Read the model definition and answer for the solid it produces. Units are mm, in the model's axes. A direction names the side the tool comes from. Coordinates: 2 decimals unless noted, no trailing zeros. Order: outer loops, then holes, each group sorted by start corner. A loop starts at its lowest first (then second) coordinate and runs counter-clockwise, first axis right, second up. Notation, with made-up numbers: M 33.5,24 L 59.5,24 A11 ccw 59.5,32 Z; hole C 78.5,14 d2. An arc over 180 degrees is marked long. One line per question, with ' | ' between items. Start each with the question number.
1) A tool of negligible diameter and unlimited length cuts with its end or side. For faces 4 (the face through (-35.357, 48.514, -99.555)), 5 (the face through (-60.933, 18, -98)), 6 (the face through (-56.17, 5.03, -97.92)), from which of +Z, -Z, +X, -X, +Y, -Y can it reach the whole face along a straight path? Write none if from no direction.
2) Given P1, Ø1.6, axis at x = -35.53, z = -98.21, coming from the +Y side; P2, Ø1.5, axis at y = -4, z = -98, coming from the +X side; P3, Ø1.6, axis at y = 6.35, z = -98.21, coming from the +X side, each flat-ended and moving along its own axis, determine where each tip first touches the part or whether it passes through.
3) Find section B-B, the plane y = 0. Write down the section's boundary in (x, z).
4) Find section D-D, the plane x = 25. Write down the section's boundary in (y, z) (3 decimals), plus the area to 3 significant figures.
5) Find section A-A, the plane x = 0. Write down the section's boundary in (y, z) (1 decimal), plus the area to 3 significant figures.
6) Find section C-C, the plane x = -39. Write down the section's boundary in (y, z) (3 decimals).
7) Consider probe 1 along X at (y, z) = (24.5, -97); probe 2 along Z at (x, y) = (-55.25, 6.35); probe 3 along X at (y, z) = (1, -99.75). Determine where each line is inside the solid, lowest interval first.
8) The mould has two halves that part along X. Classify faces 1 (the face through (-35.56, 43.21, -98.45)), 2 (the face through (-14, 53.278, -98)), 3 (the face through (34.354, 31, -98)): +X half, -X half, draft (parallel to the pull), parting line (faces both ways), or undercut.
from build123d import *

# Parameters (mm, degrees)
SKETCH1_W                 = 95.287460045
SKETCH1_H                 = 69.153467802
SKETCH1_R                 = 7.9375
BOSS_EXTRUDE1_DEPTH       = 6.35
FILLET1_R                 = 25.4
F_6_32_TAPPED_HOLE1_D     = 2.7051
F_6_32_TAPPED_HOLE1_DEPTH = 10.9728
F_6_32_TAPPED_HOLE1_TIP   = 0.81269403
F_6_32_TAPPED_HOLE2_D     = 2.7051
F_6_32_TAPPED_HOLE2_DEPTH = 9.398
F_6_32_TAPPED_HOLE2_TIP   = 0.81269403
F_6_32_TAPPED_HOLE3_D     = 2.7051
F_6_32_TAPPED_HOLE3_DEPTH = 9.398
F_6_32_TAPPED_HOLE3_TIP   = 0.81269403


with BuildPart() as part:
    # Sketch1 → Boss-Extrude1 (new body)
    with BuildSketch(Plane.XY.offset(-95.039403682)):
        with Locations((-13.289407805, 18.701733901)):
            Rectangle(SKETCH1_W, SKETCH1_H)
        Circle(SKETCH1_R, mode=Mode.SUBTRACT)
        with Locations((-35.533137827, 0)):
            Circle(SKETCH1_R, mode=Mode.SUBTRACT)
    extrude(amount=-BOSS_EXTRUDE1_DEPTH)

    # Fillet1
    fillet1_edges = [part.edges().sort_by_distance(p)[0] for p in [
        (34.354322218, -15.875, -98.214403682),
    ]]
    fillet(fillet1_edges, radius=FILLET1_R)

    # #6-32 Tapped Hole1
    with Locations(Plane.XY.offset(-95.039403682)):
        with Locations((27.559822218, 24.703467802), (3.048822218, 24.703467802)):
            Hole(F_6_32_TAPPED_HOLE1_D / 2, depth=F_6_32_TAPPED_HOLE1_DEPTH)
            with Locations((0, 0, -(F_6_32_TAPPED_HOLE1_DEPTH + F_6_32_TAPPED_HOLE1_TIP / 2))):  # 118° drill point
                Cone(0, F_6_32_TAPPED_HOLE1_D / 2, F_6_32_TAPPED_HOLE1_TIP, mode=Mode.SUBTRACT)

    # #6-32 Tapped Hole2
    with Locations(Plane(origin=(0, 53.278467802, 0), x_dir=(1, 0, 0), z_dir=(0, 1, 0))):
        with Locations((-35.533137827, 98.214403682), (2.604322218, 98.214403682)):
            Hole(F_6_32_TAPPED_HOLE2_D / 2, depth=F_6_32_TAPPED_HOLE2_DEPTH)
            with Locations((0, 0, -(F_6_32_TAPPED_HOLE2_DEPTH + F_6_32_TAPPED_HOLE2_TIP / 2))):  # 118° drill point
                Cone(0, F_6_32_TAPPED_HOLE2_D / 2, F_6_32_TAPPED_HOLE2_TIP, mode=Mode.SUBTRACT)

    # #6-32 Tapped Hole3
    with Locations(Plane.ZY.offset(60.933137827)):
        with Locations((-98.214403682, 45.340967802), (-98.214403682, 6.35)):
            Hole(F_6_32_TAPPED_HOLE3_D / 2, depth=F_6_32_TAPPED_HOLE3_DEPTH)
            with Locations((0, 0, -(F_6_32_TAPPED_HOLE3_DEPTH + F_6_32_TAPPED_HOLE3_TIP / 2))):  # 118° drill point
                Cone(0, F_6_32_TAPPED_HOLE3_D / 2, F_6_32_TAPPED_HOLE3_TIP, mode=Mode.SUBTRACT)


solid = part.part
Report:
1) face 4: +Y | face 5: +Z, -Z, -X, +Y, -Y | face 6: -X
2) P1: stops at y = 43.55 | P2: stops at x = 30.91 | P3: stops at x = 34.24
3) outline: M -60.93,-101.39 L -43.47,-101.39 L -43.47,-95.04 L -60.93,-95.04 Z; M -27.6,-101.39 L -7.94,-101.39 L -7.94,-95.04 L -27.6,-95.04 Z; M 7.94,-101.39 L 32.5,-101.39 L 32.5,-95.04 L 7.94,-95.04 Z
4) outline: M -10.165,-101.389 L 53.278,-101.389 L 53.278,-95.039 L -10.165,-95.039 Z | area: 403 mm^2
5) outline: M -15.9,-101.4 L -7.9,-101.4 L -7.9,-95 L -15.9,-95 Z; M 7.9,-101.4 L 53.3,-101.4 L 53.3,-95 L 7.9,-95 Z | area: 338 mm^2
6) outline: M -15.875,-101.389 L -7.14,-101.389 L -7.14,-95.039 L -15.875,-95.039 Z; M 7.14,-101.389 L 53.278,-101.389 L 53.278,-95.039 L 7.14,-95.039 Z
7) probe 1: x = -60.93 to 1.71, 4.39 to 26.22, 28.9 to 34.35 | probe 2: z = -101.39 to -99.57, -96.86 to -95.04 | probe 3: x = -60.93 to -43.41, -27.66 to -7.87, 7.87 to 32.88
8) face 1: undercut | face 2: draft | face 3: +X half
